Study the drawing (mm; zero at the part's minimum x, y, z) and answer. A direction names the side the tool comes from. Round coordinates to 2 decimals unless told otherwise and drop trailing zeros. Write each loop counter-clockwise with the first axis right and the second up, starting at its lowest first coordinate (ties: lowest second). Pieces come first, ordered by that corner, then holes. Notation, with made-up numbers: (0.25, 4.5) -> (32.25, 4.5) arc R16 ccw to (32.25, 14.5) -> close; hole circle Ø8 at (-7, 83). An arc over 180 degrees is marked (long way). Return JSON: item names as keys, results as strings.
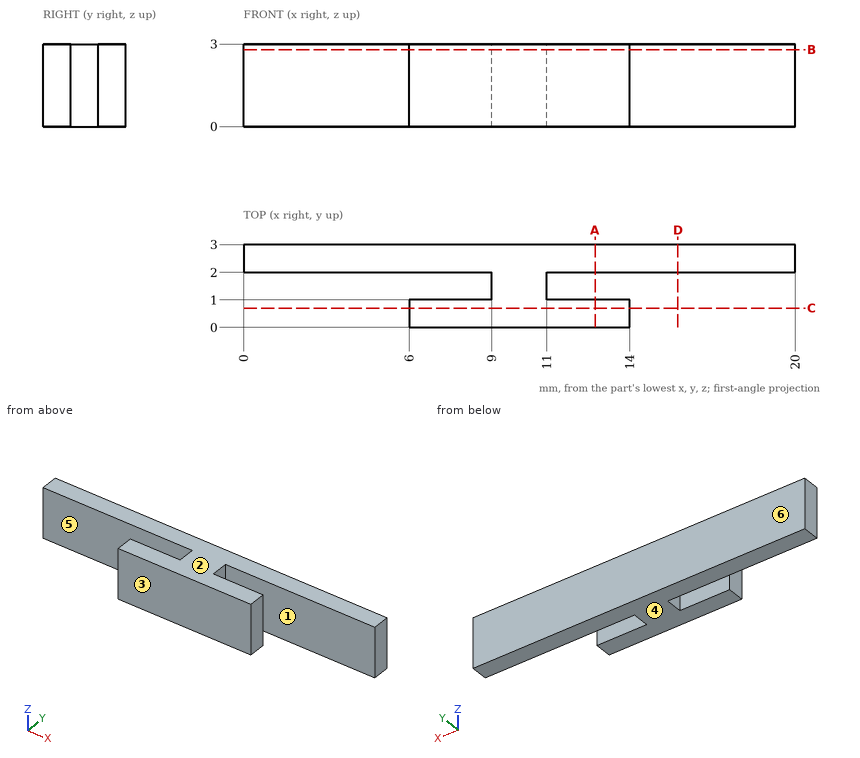
Item 1: Section B-B (z = 2.8) is taken. Give the vertices of the cut face in (x, y), then the cut area to 3 significant figures.
Worked answers:
{"outline": "(0, 2) -> (9, 2) -> (9, 1) -> (6, 1) -> (6, 0) -> (14, 0) -> (14, 1) -> (11, 1) -> (11, 2) -> (20, 2) -> (20, 3) -> (0, 3) -> close", "area": "30.0 mm2"}
Item 2: For a pull along Y with two mould halves and no side action, classify the marked faces 3, 4, 5 and 6 as released by +Y, released by -Y, zero draft, split by the parting line, or undercut.
Worked answers:
{"face 3": "released by -Y", "face 4": "zero draft", "face 5": "undercut", "face 6": "released by +Y"}
Item 3: Straight lines are drawn through the part: L1, parallel to Y at x = 7.25, z = 0.35; L2, parallel to X at y = 0.4, z = 2.4; L3, parallel to Y at x = 5.75, z = 2.6. For each, find the intervals that lie inside material, in ascending order. Write a range as [from, to].
Worked answers:
{"L1": "y = [0, 1], [2, 3]", "L2": "x = [6, 14]", "L3": "y = [2, 3]"}
Item 4: Section C-C (y = 0.7) is taken. Give the vertices of the cut face in (x, z), then the cut area to 3 significant figures.
Worked answers:
{"outline": "(6, 0) -> (14, 0) -> (14, 3) -> (6, 3) -> close", "area": "24.0 mm2"}
Item 5: Section D-D (x = 15.75) is taken. Give the vertices of the cut face in (y, z), then the cut area to 3 significant figures.
Worked answers:
{"outline": "(2, 0) -> (3, 0) -> (3, 3) -> (2, 3) -> close", "area": "3.00 mm2"}
Item 6: Section A-A (x = 12.75) is taken. Give the vertices of the cut face in (y, z).
Worked answers:
{"outline": "(0, 0) -> (1, 0) -> (1, 3) -> (0, 3) -> close; (2, 0) -> (3, 0) -> (3, 3) -> (2, 3) -> close"}
Item 7: A tool of negligible diameter and unlimited length cuts with its end or side. For the marked faces 1 and 2, from which of +Z, -Z, +X, -X, +Y, -Y can it reach the whole face along a straight path? Write none if from no direction.
Worked answers:
{"face 1": "+Z, -Z, +X", "face 2": "+Z, +X, -X, +Y, -Y"}
